from build123d import *

# Parameters (mm, degrees)
GRUNDK_RPER_DEPTH               = 100
SCHRAEGEN_VORNE_DEPTH           = 100
SCHNITT_LINEAR_AUSTRAGEN4_DEPTH = 45
WANDUNG1_T                      = -1.75


with BuildPart() as part:
    # Skizze1 → Grundkörper (new body)
    with BuildSketch(Plane.XY):
        Polygon((0, 0), (100, 0), (85, 45), (15, 45), align=None)
    extrude(amount=-GRUNDK_RPER_DEPTH)

    # Skizze2 → Schraegen_vorne (cut)
    with BuildSketch(Plane(origin=(0, 0, 0), x_dir=(0, 0, -1), z_dir=(1, 0, 0))):
        Polygon((100, 0), (87, 45), (100, 45), align=None)
    schraegen_vorne = extrude(amount=SCHRAEGEN_VORNE_DEPTH, mode=Mode.SUBTRACT)

    # Spiegel_Schraege_hinten: Schraegen_vorne across plane
    add(schraegen_vorne.mirror(Plane.XY.offset(-50)), mode=Mode.SUBTRACT)

    # Skizze4 → Schnitt-Linear austragen4 (cut)
    with BuildSketch(Plane.XZ):
        Polygon((5, 0), (95, 0), (75, -40), (25, -40), align=None)
    extrude(amount=-SCHNITT_LINEAR_AUSTRAGEN4_DEPTH, mode=Mode.SUBTRACT)

    # Skizze6 → Schnitt-Rotation1 (revolve, cut)
    with BuildSketch(Plane.ZY.offset(-50), mode=Mode.PRIVATE) as schnitt_rotation1_sk:
        with BuildLine():
            Line((-55, 20), (-40, 20))
            Line((-40, 20), (-40, 5))
            ThreePointArc((-40, 5), (-50.606601718, 9.393398282), (-55, 20))
        make_face()
    revolve(schnitt_rotation1_sk.sketch.rotate(Axis((50, 20, -127.890936505), (0, 0, 1)), 180), axis=Axis((50, 20, -127.890936505), (0, 0, 1)), mode=Mode.SUBTRACT)

    # Wandung1
    wandung1_openings = [part.faces().sort_by_distance(p)[0] for p in [
        (50, 0, -62.407407407),
    ]]
    offset(amount=WANDUNG1_T, openings=wandung1_openings, kind=Kind.INTERSECTION)


solid = part.part
For this review, take the finished solid that the model builds, in its own axes (mm). A direction names the side the tool comes from. Round coordinates to 2 decimals unless told otherwise and drop trailing zeros. Loops run counter-clockwise (first coordinate to the right, second up) from the corner with the lowest first, then second, coordinate; pieces in that order, holes last. Notation, with made-up numbers: (23, -7) - (77, -7) arc R10 ccw to (77, 8) - close; hole circle Ø5 at (-4, -19.75). An arc over 180 degrees is marked (long way). Answer as CSV lines item,"result".
(1) Mouldability with a two-part tool opening along X and no side actions: class faces 5 (the face through (49.33, 21.32, -92.02)), 6 (the face through (95.241, 9.252, -2.673)), 7 (the face through (92.6, 22.2, -49.3)) as +X half, -X half, draft (parallel to the pull), parting line (faces both ways), or undercut.
Checked values:
face 5,"undercut"
face 6,"draft"
face 7,"+X half"
(2) Tool access review of faces 1 (the face through (24, 0, -39)), 2 (the face through (83.985, 16.517, -25.943)), 3 (the face through (56, 36, -41.75)), 4 (the face through (83, 22, -24)): name each direction out of +Z, -Z, +X, -X, +Y, -Y from which nothing blocks a thin tool from reaching the whole face with its end or side.
Checked values:
face 1,"+Z, -Z, +X, -X, -Y"
face 2,"-Y"
face 3,"none"
face 4,"+Z, +Y, -Y"
(3) Consider section B-B on z = -11.5. Give the boundary of the cut face in (x, y).
Checked values:
outline,"(0, 0) - (1.84, 0) - (8.79, 20.85) - (8.79, 0) - (10.75, 0) - (10.75, 32.25) - close; (89.25, 0) - (91.21, 0) - (91.21, 20.85) - (98.16, 0) - (100, 0) - (89.25, 32.25) - close"
(4) Consider section A-A on z = -46.5. Give the boundary of the cut face in (x, y).
Checked values:
outline,"(0, 0) - (1.84, 0) - (16.26, 43.25) - (83.74, 43.25) - (98.16, 0) - (100, 0) - (85, 45) - (15, 45) - close; circle Ø30.87 at (50, 20); hole circle Ø27.04 at (50, 20)"
(5) Wall thickness on line 1 (X direction, y = 3.5, z = -14); line 2 (X direction, y = 15, z = -36); line 3 (Y direction, x = 60, z = -48.5): over which ranges is each line inside the solid? List them lowest first.
Checked values:
line 1,"x = 1.17 to 3.01, 10.04 to 12, 88 to 89.96, 96.99 to 98.83"
line 2,"x = 5 to 6.84, 21.04 to 23, 77 to 78.96, 93.16 to 95"
line 3,"y = 9.59 to 12.74, 27.26 to 30.41, 43.25 to 45"
(6) Consider section D-D on x = 69.5. Give the boundary of the cut face in (y, z), then the cut area to 3 significant figures.
Checked values:
outline,"(0, -100) - (45, -87) - (45, -40) - (0, -40) - (0, -41.75) - (43.25, -41.75) - (43.25, -85.68) - (0, -98.18) - close"
area,"237 mm2"
(7) Insertion check: P1, Ø1, axis at y = 19, z = -66.5, coming from the +X side; P2, Ø13.5, axis at x = 48.5, y = 20, coming from the +Z side; P3, Ø5, axis at y = 35.5, z = -67.5, coming from the -X side; P4, Ø6, axis at x = 13, z = -72.5, coming from the +Y side. Each pin has a flat end and moves straight along its axis. Give the tip position at first contact, or say it passes through.
Checked values:
P1,"stops at x = 93.83"
P2,"stops at z = -52.53"
P3,"stops at x = 11"
P4,"stops at y = 45"
(8) Consider section C-C on y = 18. Give the boundary of the cut face in (x, z), then the cut area to 3 significant figures.
Checked values:
outline,"(6, -94.8) - (94, -94.8) - (94, -5.2) - (92.4, -5.2) - (75, -40) - (64.87, -40) arc R14.87 cw to (35.13, -40) - (25, -40) - (7.6, -5.2) - (6, -5.2) - close; hole (7.84, -92.98) - (92.16, -92.98) - (92.16, -9.6) - (76.08, -41.75) - (66.54, -41.75) arc R16.63 cw to (33.46, -41.75) - (23.92, -41.75) - (7.84, -9.6) - close"
area,"733 mm2"
